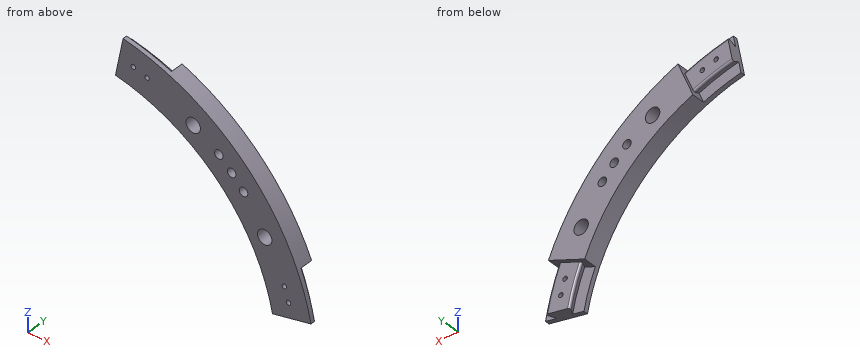
```python
from build123d import *

# Parameters (mm, degrees)
SKETCH1_W                = 28.575
SKETCH1_H                = 12.7
CUT_EXTRUDE1_DEPTH       = 9.525
F_12_CLEARANCE_HOLE1_D   = 6.2484
M4X0_7_TAPPED_HOLE1_D    = 3.3
CIRPATTERN1_COUNT        = 4
Z_0_413_DIAMETER_HOLE1_D = 10.4902
FILLET1_R                = 1.27
CUT_EXTRUDE2_DEPTH       = 247.298196718
CUT_EXTRUDE2_DEPTH_BACK  = 247.298196718


with BuildPart() as part:
    # Sketch1 → Revolve1 (revolve)
    with BuildSketch(Plane.XY, mode=Mode.PRIVATE) as revolve1_sk:
        with Locations((159.813733777, 1058.545)):
            Rectangle(SKETCH1_W, SKETCH1_H)
    revolve(revolve1_sk.sketch.rotate(Axis((0, 1125.81516809, 0), (0, -1, 0)), 180), axis=Axis((0, 1125.81516809, 0), (0, -1, 0)))

    # Sketch19 → Cut-Extrude1 (cut)
    with BuildSketch(Plane(origin=(0, 1064.895, 0), x_dir=(1, 0, 0), z_dir=(0, 1, 0))):
        with BuildLine():
            Line((160.848566471, -66.625657721), (134.44870883, -55.690478641))
            ThreePointArc((134.44870883, -55.690478641), (145.526233777, 0), (134.44870883, 55.690478641))
            Line((134.44870883, 55.690478641), (160.848566471, 66.625657721))
            ThreePointArc((160.848566471, 66.625657721), (174.101233777, 0), (160.848566471, -66.625657721))
        make_face()
        with BuildLine():
            Line((-66.625657721, 160.848566471), (-55.690478641, 134.44870883))
            ThreePointArc((-55.690478641, 134.44870883), (0, 145.526233777), (55.690478641, 134.44870883))
            Line((55.690478641, 134.44870883), (66.625657721, 160.848566471))
            ThreePointArc((66.625657721, 160.848566471), (0, 174.101233777), (-66.625657721, 160.848566471))
        make_face()
        with BuildLine():
            Line((-134.44870883, -55.690478641), (-160.848566471, -66.625657721))
            ThreePointArc((-160.848566471, -66.625657721), (-174.101233777, 0), (-160.848566471, 66.625657721))
            Line((-160.848566471, 66.625657721), (-134.44870883, 55.690478641))
            ThreePointArc((-134.44870883, 55.690478641), (-145.526233777, 0), (-134.44870883, -55.690478641))
        make_face()
        with BuildLine():
            Line((-55.690478641, -134.44870883), (-66.625657721, -160.848566471))
            ThreePointArc((-66.625657721, -160.848566471), (0, -174.101233777), (66.625657721, -160.848566471))
            Line((66.625657721, -160.848566471), (55.690478641, -134.44870883))
            ThreePointArc((55.690478641, -134.44870883), (0, -145.526233777), (-55.690478641, -134.44870883))
        make_face()
    extrude(amount=-CUT_EXTRUDE1_DEPTH, mode=Mode.SUBTRACT)

    # Sketch21 → Revolve2 (revolve)
    with BuildSketch(Plane.XY):
        Polygon((-165.672559567, 1055.37), (-153.954907986, 1055.37), (-150.288733777, 1061.72), (-169.338733777, 1061.72), align=None)
    revolve(axis=Axis((0, 0, 0), (0, 1, 0)))

    # #12 Clearance Hole1 (through all)
    with Locations(Plane(origin=(0, 1052.195, 0), x_dir=(-1, 0, 0), z_dir=(0, -1, 0))):
        with Locations((103.667734326, 121.628246568), (121.628246568, 103.667734326), (113.00537488, 113.00537488)):
            f_12_clearance_hole1 = Hole(F_12_CLEARANCE_HOLE1_D / 2)

    # M4x0.7 Tapped Hole1 (through all)
    with Locations(Plane(origin=(0, 1061.72, 0), x_dir=(1, 0, 0), z_dir=(0, 1, 0))):
        with Locations((-51.370441133, 151.33243962), (-41.36283797, 154.36821285), (51.370441133, 151.33243962), (41.36283797, 154.36821285)):
            m4x0_7_tapped_hole1 = Hole(M4X0_7_TAPPED_HOLE1_D / 2)

    # CirPattern1: #12 Clearance Hole1, M4x0.7 Tapped Hole1 ×4 about axis
    cirpattern1_axis = Axis((0, 0, 0), (0, 1, 0))
    add([f_12_clearance_hole1.rotate(cirpattern1_axis, i * 360 / CIRPATTERN1_COUNT) for i in range(1, CIRPATTERN1_COUNT)], mode=Mode.SUBTRACT)
    add([m4x0_7_tapped_hole1.rotate(cirpattern1_axis, i * 360 / CIRPATTERN1_COUNT) for i in range(1, CIRPATTERN1_COUNT)], mode=Mode.SUBTRACT)

    # Z (0.413) Diameter Hole1 (through all)
    with Locations(Plane(origin=(0, 1064.895, 0), x_dir=(1, 0, 0), z_dir=(0, 1, 0))):
        with Locations((-137.027937996, -79.113116888), (137.027937996, -79.113116888), (137.027937996, 79.113116888), (-137.027937996, 79.113116888), (-85.014893438, 133.44665207), (85.014893438, 133.44665207), (85.014893438, -133.44665207), (-85.014893438, -133.44665207)):
            Hole(Z_0_413_DIAMETER_HOLE1_D / 2)

    # Fillet1
    fillet1_edges = [part.edges().sort_by_distance(p)[0] for p in [
        (-150.288733777, 1061.72, 0),
        (0, 1061.72, 150.288733777),
        (0, 1061.72, -150.288733777),
        (150.288733777, 1061.72, 0),
        (-169.338733777, 1061.72, 0),
        (0, 1061.72, 169.338733777),
        (0, 1061.72, -169.338733777),
        (169.338733777, 1061.72, 0),
    ]]
    fillet(fillet1_edges, radius=FILLET1_R)

    # Sketch23 → Cut-Extrude2 (cut, two sides: drawn at the far end of the back side and taken through both)
    with BuildSketch(Plane(origin=(0, 1058.545, 0), x_dir=(1, 0, 0), z_dir=(0, 1, 0)).offset(-CUT_EXTRUDE2_DEPTH_BACK)):
        with BuildLine():
            ThreePointArc((174.101233777, 0), (173.262888749, 17.064905063), (170.755927388, 33.965465761))
            Line((170.755927388, 33.965465761), (142.729988001, 28.390759809))
            ThreePointArc((142.729988001, 28.390759809), (144.825485185, 14.264065278), (145.526233777, 0))
            ThreePointArc((145.526233777, 0), (144.825485185, -14.264065278), (142.729988001, -28.390759809))
            Line((142.729988001, -28.390759809), (170.755927388, -33.965465761))
            ThreePointArc((170.755927388, -33.965465761), (173.262888749, -17.064905063), (174.101233777, 0))
        make_face()
        with BuildLine():
            Line((-142.729988001, 28.390759809), (-170.755927388, 33.965465761))
            ThreePointArc((-170.755927388, 33.965465761), (-174.101233777, 0), (-170.755927388, -33.965465761))
            Line((-170.755927388, -33.965465761), (-142.729988001, -28.390759809))
            ThreePointArc((-142.729988001, -28.390759809), (-145.526233777, 0), (-142.729988001, 28.390759809))
        make_face()
        with BuildLine():
            Line((28.390759809, 142.729988001), (33.965465761, 170.755927388))
            ThreePointArc((33.965465761, 170.755927388), (0, 174.101233777), (-33.965465761, 170.755927388))
            Line((-33.965465761, 170.755927388), (-28.390759809, 142.729988001))
            ThreePointArc((-28.390759809, 142.729988001), (0, 145.526233777), (28.390759809, 142.729988001))
        make_face()
        with BuildLine():
            ThreePointArc((28.390759809, -142.729988001), (0, -145.526233777), (-28.390759809, -142.729988001))
            Line((-28.390759809, -142.729988001), (-33.965465761, -170.755927388))
            ThreePointArc((-33.965465761, -170.755927388), (0, -174.101233777), (33.965465761, -170.755927388))
            Line((33.965465761, -170.755927388), (28.390759809, -142.729988001))
        make_face()
    extrude(amount=CUT_EXTRUDE2_DEPTH + CUT_EXTRUDE2_DEPTH_BACK, mode=Mode.SUBTRACT)


with BuildPart() as cut_extrude2_kept_piece:
    # of the separate pieces the step leaves, the one the design keeps (cut_extrude2_pieces_kept)
    add(part.part.solids().sort_by_distance((32.321112995, 1055.37, 162.48920779))[0])


solid = cut_extrude2_kept_piece.part
```
Read the model definition and answer for the solid it produces. Units are mm, in the model's axes. Round coordinates to 2 decimals unless told otherwise and drop trailing zeros. Write each loop counter-clockwise with the first axis right and the second up, starting at its lowest first coordinate (ties: lowest second). Pieces come first, ordered by that corner, then holes. Notation, with made-up numbers: (60.5, 1.5) -> (119.5, 1.5) arc R10 ccw to (119.5, 19.5) -> close; hole circle Ø4 at (38, -14.75). An arc over 180 degrees is marked (long way). Answer in a Markdown table with one row per item. Add a question column.
1) Consider line 1 (Y direction, x = 60, z = 159.5) (3 decimals); line 2 (Z direction, x = 154, y = 1057.25); line 3 (Z direction, x = 40.5, y = 1060). Determine where each line is inside the solid, lowest interval first.
2) Given P1, Ø14, axis at x = 50, z = 166, coming from the +Y side; P2, Ø4, axis at x = 62.5, y = 1057, coming from the -Z side; P3, Ø3.5, axis at x = 121.63, z = 103.67, coming from the +Y side; P4, Ø1.5, axis at y = 1056, z = 86, coming from the -X side, each flat-ended and moving along its own axis, determine where each tip first touches the part or whether it passes through.
3) Find section B-B, the plane x = 97.5. Determine the outline of the cut face in (y, z) (3 decimals).
4) Find section A-A, the plane y = 1057. State how many separate pieces and enclosed holes the cut face has, and give its area (3 significant figures).
5) Find section C-C, the plane z = 94.5. Determine the outline of the cut face in (x, y) (3 decimals).
Findings below:
| question | item | result |
|---|---|---|
| 1 | line 1 | 1052.195 to 1055.37 |
| 1 | line 2 | 30.63 to 39.75, 42.97 to 81.21 |
| 1 | line 3 | 145.78 to 152.96, 155.77 to 163.38 |
| 2 | P1 | y = 1061.72 |
| 2 | P2 | z = 130.45 |
| 2 | P3 | through |
| 2 | P4 | x = 116.84 |
| 3 | outline | (1052.195, 108.035) -> (1064.895, 108.035) -> (1064.895, 144.239) -> (1052.195, 144.239) -> close |
| 4 | separate pieces | 1 |
| 4 | enclosed holes | 9 |
| 4 | area | 4,140 mm² |
| 5 | outline | (110.669, 1052.195) -> (146.222, 1052.195) -> (146.222, 1064.895) -> (110.669, 1064.895) -> close |
